```python
from build123d import *

# Parameters (mm, degrees)
F0_R     = 9.525
F1_DEPTH = 9.525


with BuildPart() as f1:
    # F0 (on Right) → F1 (new body)
    with BuildSketch(Plane.YZ):
        Polygon((50.8, 25.4), (-50.8, 25.4), (-50.8, -25.4), (38.320067, -25.4), (42.387699, -25.4), (50.8, -25.4), align=None)
        with Locations((-35.469551, -12.90859)):
            Circle(F0_R, mode=Mode.SUBTRACT)
        with Locations((38.260598, -13.141178)):
            Circle(F0_R, mode=Mode.SUBTRACT)
        with Locations((-35.469551, 13.141178)):
            Circle(F0_R, mode=Mode.SUBTRACT)
        with Locations((36.865074, 11.745654)):
            Circle(F0_R, mode=Mode.SUBTRACT)
        with BuildLine():
            Line((42.387699, -25.4), (38.320067, -25.4))
            ThreePointArc((38.320067, -25.4), (40.353883, -25.619667), (42.387699, -25.4))
        make_face()
    extrude(amount=F1_DEPTH)


solid = f1.part
```
Build history of the part. All positions in model axes, mm. A direction names the side the tool comes from. Round coordinates to 2 decimals unless told otherwise and drop trailing zeros. Loops run counter-clockwise (first coordinate to the right, second up) from the corner with the lowest first, then second, coordinate; pieces in that order, holes last.
Item 1: Drill centre lines: line 1 along Y through (x, z) = (2, -13.5); line 2 along Y through (x, z) = (6.5, -19); line 3 along Z through (x, y) = (1, -37). Where is each one in solid material? Low to high.
Item 2: Two-plate mould, pull along Z, no slides. Class faces 1 (the face through (5, 50.8, 0)), 2 (the face through (5, 47, -25.4)), 3 (the face through (4.7, 29.84, 18.18)): released by +Z, released by -Z, zero draft, split by the parting line, or undercut.
Item 3: Saw through at C-C (z = 6). List the corners of the cut face in (x, y) (3 decimals).
Item 4: Pin check, flat tip, straight feed: P1, Ø5, axis at x = 7.5, y = 35, coming from the -Z side. Stop position of the tip, or through.
Item 5: Which spindle directions (+Z, -Z, +X, -X, +Y, -Y) get a long thin tool onto all of the face, cutting with end or side? Do faces 4 (the face through (5, -7, -25.4)), 5 (the face through (5, 1, 25.4)). Say none if no direction does.
Item 6: Saw through at A-A (y = -33). List the corners of the cut face in (x, z) (3 decimals), then the cut area to 3 significant figures.
Item 7: Saw through at B-B (x = 3.5). List the corners of the cut face in (y, z) (3 decimals), then the cut area to 3 significant figures.
Worked answers:
1. line 1: y = -50.8 to -44.98, -25.96 to 28.74, 47.78 to 50.8
1. line 2: y = -50.8 to -42.79, -28.15 to 30.75, 45.77 to 50.8
1. line 3: z = -25.4 to -22.31, -3.51 to 3.74, 22.54 to 25.4
2. face 1: zero draft
2. face 2: released by -Z
2. face 3: undercut
3. outline: (0, -50.8) - (9.525, -50.8) - (9.525, -41.773) - (0, -41.773) - close; (0, -29.166) - (9.525, -29.166) - (9.525, 29.268) - (0, 29.268) - close; (0, 44.462) - (9.525, 44.462) - (9.525, 50.8) - (0, 50.8) - close
4. P1: stops at z = -25.4
5. face 4: -Z, +X, -X, -Y
5. face 5: +Z, +X, -X, +Y, -Y
6. outline: (0, -25.4) - (9.525, -25.4) - (9.525, -22.108) - (0, -22.108) - close; (0, -3.709) - (9.525, -3.709) - (9.525, 3.942) - (0, 3.942) - close; (0, 22.34) - (9.525, 22.34) - (9.525, 25.4) - (0, 25.4) - close
6. area: 133 mm2
7. outline: (-50.8, -25.4) - (38.32, -25.4) arc R9.525 ccw to (42.388, -25.4) - (50.8, -25.4) - (50.8, 25.4) - (-50.8, 25.4) - close; hole circle Ø19.05 at (-35.47, -12.909); hole circle Ø19.05 at (-35.47, 13.141); hole circle Ø19.05 at (36.865, 11.746); hole circle Ø19.05 at (38.261, -13.141)
7. area: 4,020 mm2
